Geometry: final body of the model. Coordinates: model frame, mm. Face numbers are marked on the shaded views. A direction names the side the tool comes from. Round coordinates to 2 decimals unless told otherwise and drop trailing zeros. Loops run counter-clockwise (first coordinate to the right, second up) from the corner with the lowest first, then second, coordinate; pieces in that order, holes last. Notation, with made-up numbers: M 18,48 L 54,48 A30 cw 54,72 Z; hole C 75.5,-3 d11. An arc over 180 degrees is marked long. Answer as a JSON object with one key per item and string values.
```python
from build123d import *

# Parameters (mm, degrees)
F1_DEPTH = 60
F2_R     = 5
F3_SIZE  = 5
F4_R     = 25.516517
F5_DEPTH = 30


with BuildPart() as f1:
    # F0 (on Front) → F1 (new body)
    with BuildSketch(Plane.XZ):
        with BuildLine():
            Line((40.062132, 48.475344), (-33.937868, 48.475344))
            Line((-33.937868, 48.475344), (-46.937868, 35.475344))
            Line((-46.937868, 35.475344), (-46.937868, -36.524656))
            ThreePointArc((-46.937868, -36.524656), (-42.544469, -47.131258), (-31.937868, -51.524656))
            Line((-31.937868, -51.524656), (40.062132, -51.524656))
            Line((40.062132, -51.524656), (53.062132, -38.524656))
            Line((53.062132, -38.524656), (53.062132, 35.475344))
            ThreePointArc((53.062132, 35.475344), (49.25452, 44.667732), (40.062132, 48.475344))
        make_face()
    extrude(amount=F1_DEPTH)

    # F2
    f2_edges = [f1.edges().sort_by_distance(p)[0] for p in [
        (3.062132, -60, 48.475344),
        (-40.437868, -60, 41.975344),
        (-46.937868, -60, -0.524656),
        (-42.544469, -60, -47.131258),
        (4.062132, -60, -51.524656),
        (46.562132, -60, -45.024656),
        (53.062132, -60, -1.524656),
        (49.25452, -60, 44.667732),
    ]]
    fillet(f2_edges, radius=F2_R)

    # F3
    f3_edges = [f1.edges().sort_by_distance(p)[0] for p in [
        (3.062132, 0, 48.475344),
        (-40.437868, 0, 41.975344),
        (-46.937868, 0, -0.524656),
        (-42.544469, 0, -47.131258),
        (4.062132, 0, -51.524656),
        (46.562132, 0, -45.024656),
        (53.062132, 0, -1.524656),
        (49.25452, 0, 44.667732),
    ]]
    chamfer(f3_edges, length=F3_SIZE)

    # F4 (on face) → F5 (cut)
    with BuildSketch(Plane.XZ.offset(60)):
        with Locations((2.964985, 0)):
            Circle(F4_R)
    extrude(amount=-F5_DEPTH, mode=Mode.SUBTRACT)


solid = f1.part
```
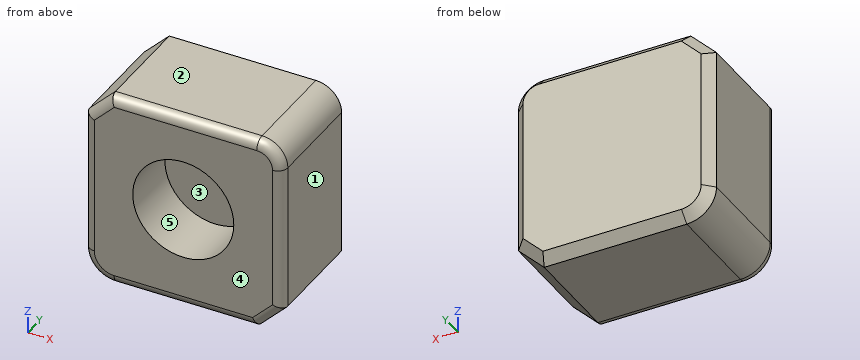
1) Set-up query: the marked faces 4 and 5. Return all of +Z, -Z, +X, -X, +Y, -Y with unobstructed straight access to the full face (end or side cutting, diameter ignored); none if empty.
Geometry results:
{"face 4": "+Z, -Z, +X, -X, -Y", "face 5": "-Y"}
2) Cut plane B-B on y = -22.5. Return the cut outline in (x, z), and give its area (3 significant figures).
Geometry results:
{"outline": "M -46.94,-36.52 A15 ccw -31.94,-51.52 L 40.06,-51.52 L 53.06,-38.52 L 53.06,35.48 A13 ccw 40.06,48.48 L -33.94,48.48 L -46.94,35.48 Z", "area": "9,750 mm2"}
3) First-contact query: pin 1 (1.5 mm diameter, centred on y = -47.5, z = -40.5, fed in from +X). Flat tip, straight axial feed; report the tip coordinate or a pass-through.
Geometry results:
{"pin 1": "x = 51.84"}
4) Pull-direction query (Z, two-part tool) for the marked faces 1, 2 and 3; classes: +Z half, -Z half, draft (parallel to the pull), parting line (faces both ways), or undercut.
Geometry results:
{"face 1": "draft", "face 2": "+Z half", "face 3": "undercut"}
5) Cut plane C-C on x = 27. Return the cut outline in (y, z).
Geometry results:
{"outline": "M -60,-46.52 A5 ccw -55,-51.52 L -5,-51.52 L 0,-46.52 L 0,43.48 L -5,48.48 L -55,48.48 A5 ccw -60,43.48 L -60,8.57 L -30,8.57 L -30,-8.57 L -60,-8.57 Z"}
6) Cut plane A-A on z = 0. Return the cut outline in (x, y), and give its area (3 significant figures).
Geometry results:
{"outline": "M -46.94,-55 A5 ccw -41.94,-60 L -22.55,-60 L -22.55,-30 L 28.48,-30 L 28.48,-60 L 48.06,-60 A5 ccw 53.06,-55 L 53.06,-5 L 48.06,0 L -41.94,0 L -46.94,-5 Z", "area": "4,430 mm2"}
7) Line query: probe 1 along X at (y, z) = (-39, 5); probe 2 along Y at (x, z) = (-18, 1); probe 3 along Z at (x, y) = (-31.5, -55.5). Output: solid intervals per line, ascending.
Geometry results:
{"probe 1": "-46.94 to -22.06, 27.99 to 53.06", "probe 2": "-30 to 0", "probe 3": "-51.5 to 48.45"}
